Geometry: final body of the model. Coordinates: model frame, mm. A direction names the side the tool comes from. Give positions to 0.01 mm unless a question says otherwise; leave off trailing zeros. Order: outer loops, then holes, each group sorted by start corner. A loop starts at its lowest first (then second) coordinate and runs counter-clockwise, first axis right, second up. Notation, with made-up numbers: (47, -29.75) - (86, -29.75) arc R15 cw to (86, -12.75) - close; hole circle Ø8 at (35.25, -23.75). An arc over 180 degrees is marked (long way). Use one line per item in the form item = value.
from build123d import *

# Parameters (mm, degrees)
F0_W     = 31.9
F0_H     = 9.57
F1_DEPTH = 7.89
F2_R     = 2.44
F3_DEPTH = 1.85
F4_R     = 1.555
F5_DEPTH = 8.38


with BuildPart() as f1:
    # F0 (on Front) → F1 (new body)
    with BuildSketch(Plane.XZ):
        with Locations((-10.049382, -0.941054)):
            Rectangle(F0_W, F0_H)
    extrude(amount=F1_DEPTH)

    # F2 (on face) → F3 (join)
    with BuildSketch(Plane.XY.offset(3.843946)):
        with Locations((-22.560522, -3.97)):
            Circle(F2_R)
        with Locations((-14.570678, -3.92)):
            Circle(F2_R)
        with Locations((-6.580835, -3.97)):
            Circle(F2_R)
        with Locations((1.409165, -3.97)):
            Circle(F2_R)
    extrude(amount=F3_DEPTH)

    # F4 (on face) → F5 (cut)
    with BuildSketch(Plane(origin=(0, 0, -5.726054), x_dir=(1, 0, 0), z_dir=(0, 0, -1))):
        with BuildLine():
            Line((-11.118799, 6.840625), (-24.567948, 6.840625))
            Line((-24.567948, 6.840625), (-24.567948, 1.076743))
            Line((-24.567948, 1.076743), (-11.118799, 1.076743))
            Line((-11.118799, 1.076743), (-11.118799, 2.733773))
            ThreePointArc((-11.118799, 2.733773), (-12.032356, 4.15031), (-11.118799, 5.566847))
            Line((-11.118799, 5.566847), (-11.118799, 6.840625))
        make_face()
        with Locations((-18.574382, 3.945)):
            Circle(F4_R, mode=Mode.SUBTRACT)
        with BuildLine():
            Line((4.891893, 6.840625), (-10.038799, 6.840625))
            Line((-10.038799, 6.840625), (-10.038799, 5.642185))
            ThreePointArc((-10.038799, 5.642185), (-9.23237, 5.081993), (-8.922356, 4.15031))
            ThreePointArc((-8.922356, 4.15031), (-9.23237, 3.218627), (-10.038799, 2.658435))
            Line((-10.038799, 2.658435), (-10.038799, 1.076743))
            Line((-10.038799, 1.076743), (4.891893, 1.076743))
            Line((4.891893, 1.076743), (4.891893, 6.840625))
        make_face()
        with Locations((-2.552682, 4.114562)):
            Circle(F4_R, mode=Mode.SUBTRACT)
    extrude(amount=-F5_DEPTH, mode=Mode.SUBTRACT)


solid = f1.part
(1) Cut plane B-B on x = -15.5. Output: boundary loops of the cut face in (y, z).
Computed values:
outline = (-7.89, -5.73) - (-6.84, -5.73) - (-6.84, 2.65) - (-1.08, 2.65) - (-1.08, -5.73) - (0, -5.73) - (0, 3.84) - (-1.66, 3.84) - (-1.66, 5.69) - (-6.18, 5.69) - (-6.18, 3.84) - (-7.89, 3.84) - close
(2) Cut plane A-A on z = -1.25. Output: boundary loops of the cut face in (x, y) (3 decimals), plus the area to 3 significant figures.
Computed values:
outline = (-25.999, -7.89) - (5.901, -7.89) - (5.901, 0) - (-25.999, 0) - close; circle Ø3.11 at (-18.574, -3.945); circle Ø3.11 at (-2.553, -4.115); hole (-24.568, -6.841) - (-11.119, -6.841) - (-11.119, -5.567) arc R1.555 cw to (-11.119, -2.734) - (-11.119, -1.077) - (-24.568, -1.077) - close; hole (-10.039, -6.841) - (4.892, -6.841) - (4.892, -1.077) - (-10.039, -1.077) - (-10.039, -2.658) arc R1.555 cw to (-8.922, -4.15) arc R1.555 cw to (-10.039, -5.642) - close
area = 108 mm²
(3) Pull-direction query (X, two-part tool) for faces 4 (the face through (-11.119, -2, -2)), 5 (the face through (-25.999, -4, -1)), 6 (the face through (-3, -4, -5.726)); classes: released by +X, released by -X, zero draft, split by the parting line, or undercut.
Computed values:
face_4 = undercut
face_5 = released by -X
face_6 = zero draft
(4) Ray query, line 1 along X through (y, z) = (-2.25, -1.5); line 2 along Y through (x, z) = (-21.5, -1); line 3 along X through (y, z) = (-5, 4). Return the intervals inside material, ascending.
Computed values:
line_1 = -26 to -24.57, -11.12 to -10.04, 4.89 to 5.9
line_2 = -7.89 to -6.84, -1.08 to 0
line_3 = -24.77 to -20.35, -16.76 to -12.38, -8.79 to -4.37, -0.8 to 3.62
(5) Cut plane C-C on y = -6. Output: boundary loops of the cut face in (x, z), plus the area to 3 significant figures.
Computed values:
outline = (-26, -5.73) - (-24.57, -5.73) - (-24.57, 2.65) - (-11.12, 2.65) - (-11.12, -5.73) - (-10.04, -5.73) - (-10.04, 2.65) - (4.89, 2.65) - (4.89, -5.73) - (5.9, -5.73) - (5.9, 3.84) - (2.76, 3.84) - (2.76, 5.69) - (0.06, 5.69) - (0.06, 3.84) - (-5.23, 3.84) - (-5.23, 5.69) - (-7.93, 5.69) - (-7.93, 3.84) - (-13.3, 3.84) - (-13.3, 5.69) - (-15.85, 5.69) - (-15.85, 3.84) - (-21.21, 3.84) - (-21.21, 5.69) - (-23.91, 5.69) - (-23.91, 3.84) - (-26, 3.84) - close
area = 87.2 mm²
(6) Reachability of faces 1 (the face through (4.892, -4, -2)), 2 (the face through (1, -4, 5.694)), 3 (the face through (-20.233, -3.237, 4.756)) from +Z, -Z, +X, -X, +Y, -Y: full face, straight path, thin tool, end or side. Return the list, or none.
Computed values:
face_1 = -Z
face_2 = +Z, +X, -X, +Y, -Y
face_3 = +Z
(7) Cut plane D-D on x = -0.5. Output: boundary loops of the cut face in (y, z), plus the area to 3 significant figures.
Computed values:
outline = (-7.89, -5.73) - (-6.84, -5.73) - (-6.84, 2.65) - (-1.08, 2.65) - (-1.08, -5.73) - (0, -5.73) - (0, 3.84) - (-2.45, 3.84) - (-2.45, 5.69) - (-5.49, 5.69) - (-5.49, 3.84) - (-7.89, 3.84) - close
area = 32.8 mm²
